from build123d import *

# Parameters (mm, degrees)
PAD_DEPTH       = 100
POCKET_DEPTH    = 2
POCKET001_DEPTH = 3


with BuildPart() as part:
    # Sketch → Pad (new body)
    with BuildSketch(Plane.XZ):
        Polygon((0, 0), (-15, 0), (-15, 1.5), (-14, 1.5), (-14, 5.5), (-17.5, 6.5), (-17.5, 7.5), (-12.5, 7.5), (-12.5, 1.5), (0, 1.5), (12.5, 1.5), (12.5, 7.5), (17.5, 7.5), (17.51485, 6.5), (14, 5.5), (14, 1.5), (15, 1.5), (15, 0), align=None)
    extrude(amount=PAD_DEPTH)

    # Sketch001 (on Face10 of Pad) → Pocket (cut)
    with BuildSketch(Plane(origin=(0, 0, 1.5), x_dir=(-1, 0, 0), z_dir=(0, 0, 1))):
        with BuildLine():
            ThreePointArc((2.5, 4.187631), (0, 6.687631), (-2.5, 4.187631))
            Line((-2.5, 4.187631), (-2.5, -0.812369))
            ThreePointArc((-2.5, -0.812369), (0, -3.312369), (2.5, -0.812369))
            Line((2.5, 4.187631), (2.5, -0.812369))
        make_face()
        with BuildLine():
            ThreePointArc((2.50462, 16.68763), (0.00462, 19.18763), (-2.49538, 16.68763))
            Line((-2.49538, 16.68763), (-2.49538, 11.68763))
            ThreePointArc((-2.49538, 11.68763), (0.00462, 9.18763), (2.50462, 11.68763))
            Line((2.50462, 16.68763), (2.50462, 11.68763))
        make_face()
        with BuildLine():
            ThreePointArc((2.509241, 29.187629), (0.009241, 31.687629), (-2.490759, 29.187629))
            Line((-2.490759, 29.187629), (-2.490759, 24.187629))
            ThreePointArc((-2.490759, 24.187629), (0.009241, 21.687629), (2.509241, 24.187629))
            Line((2.509241, 29.187629), (2.509241, 24.187629))
        make_face()
        with BuildLine():
            ThreePointArc((2.513861, 41.687629), (0.013861, 44.187629), (-2.486139, 41.687629))
            Line((-2.486139, 41.687629), (-2.486139, 36.687629))
            ThreePointArc((-2.486139, 36.687629), (0.013861, 34.187629), (2.513861, 36.687629))
            Line((2.513861, 41.687629), (2.513861, 36.687629))
        make_face()
        with BuildLine():
            ThreePointArc((2.518482, 54.187628), (0.018482, 56.687628), (-2.481518, 54.187628))
            Line((-2.481518, 54.187628), (-2.481518, 49.187628))
            ThreePointArc((-2.481518, 49.187628), (0.018482, 46.687628), (2.518482, 49.187628))
            Line((2.518482, 54.187628), (2.518482, 49.187628))
        make_face()
        with BuildLine():
            ThreePointArc((2.523102, 66.687627), (0.023102, 69.187627), (-2.476898, 66.687627))
            Line((-2.476898, 66.687627), (-2.476898, 61.687627))
            ThreePointArc((-2.476898, 61.687627), (0.023102, 59.187627), (2.523102, 61.687627))
            Line((2.523102, 66.687627), (2.523102, 61.687627))
        make_face()
        with BuildLine():
            ThreePointArc((2.527723, 79.187626), (0.027723, 81.687626), (-2.472277, 79.187626))
            Line((-2.472277, 79.187626), (-2.472277, 74.187626))
            ThreePointArc((-2.472277, 74.187626), (0.027723, 71.687626), (2.527723, 74.187626))
            Line((2.527723, 79.187626), (2.527723, 74.187626))
        make_face()
        with BuildLine():
            ThreePointArc((2.532343, 91.687625), (0.032343, 94.187625), (-2.467657, 91.687625))
            Line((-2.467657, 91.687625), (-2.467657, 86.687625))
            ThreePointArc((-2.467657, 86.687625), (0.032343, 84.187625), (2.532343, 86.687625))
            Line((2.532343, 91.687625), (2.532343, 86.687625))
        make_face()
        with BuildLine():
            ThreePointArc((2.536964, 104.187624), (0.036964, 106.687624), (-2.463036, 104.187624))
            Line((-2.463036, 104.187624), (-2.463036, 99.187624))
            ThreePointArc((-2.463036, 99.187624), (0.036964, 96.687624), (2.536964, 99.187624))
            Line((2.536964, 104.187624), (2.536964, 99.187624))
        make_face()
        with BuildLine():
            ThreePointArc((2.541584, 116.687623), (0.041584, 119.187623), (-2.458416, 116.687623))
            Line((-2.458416, 116.687623), (-2.458416, 111.687623))
            ThreePointArc((-2.458416, 111.687623), (0.041584, 109.187623), (2.541584, 111.687623))
            Line((2.541584, 116.687623), (2.541584, 111.687623))
        make_face()
    extrude(amount=-POCKET_DEPTH, mode=Mode.SUBTRACT)

    # Sketch001 (on Face10 of Pad) → Pocket001 (cut)
    with BuildSketch(Plane(origin=(0, 0, 1.5), x_dir=(-1, 0, 0), z_dir=(0, 0, 1))):
        with BuildLine():
            ThreePointArc((2.5, 4.187631), (0, 6.687631), (-2.5, 4.187631))
            Line((-2.5, 4.187631), (-2.5, -0.812369))
            ThreePointArc((-2.5, -0.812369), (0, -3.312369), (2.5, -0.812369))
            Line((2.5, 4.187631), (2.5, -0.812369))
        make_face()
        with BuildLine():
            ThreePointArc((2.50462, 16.68763), (0.00462, 19.18763), (-2.49538, 16.68763))
            Line((-2.49538, 16.68763), (-2.49538, 11.68763))
            ThreePointArc((-2.49538, 11.68763), (0.00462, 9.18763), (2.50462, 11.68763))
            Line((2.50462, 16.68763), (2.50462, 11.68763))
        make_face()
        with BuildLine():
            ThreePointArc((2.509241, 29.187629), (0.009241, 31.687629), (-2.490759, 29.187629))
            Line((-2.490759, 29.187629), (-2.490759, 24.187629))
            ThreePointArc((-2.490759, 24.187629), (0.009241, 21.687629), (2.509241, 24.187629))
            Line((2.509241, 29.187629), (2.509241, 24.187629))
        make_face()
        with BuildLine():
            ThreePointArc((2.513861, 41.687629), (0.013861, 44.187629), (-2.486139, 41.687629))
            Line((-2.486139, 41.687629), (-2.486139, 36.687629))
            ThreePointArc((-2.486139, 36.687629), (0.013861, 34.187629), (2.513861, 36.687629))
            Line((2.513861, 41.687629), (2.513861, 36.687629))
        make_face()
        with BuildLine():
            ThreePointArc((2.518482, 54.187628), (0.018482, 56.687628), (-2.481518, 54.187628))
            Line((-2.481518, 54.187628), (-2.481518, 49.187628))
            ThreePointArc((-2.481518, 49.187628), (0.018482, 46.687628), (2.518482, 49.187628))
            Line((2.518482, 54.187628), (2.518482, 49.187628))
        make_face()
        with BuildLine():
            ThreePointArc((2.523102, 66.687627), (0.023102, 69.187627), (-2.476898, 66.687627))
            Line((-2.476898, 66.687627), (-2.476898, 61.687627))
            ThreePointArc((-2.476898, 61.687627), (0.023102, 59.187627), (2.523102, 61.687627))
            Line((2.523102, 66.687627), (2.523102, 61.687627))
        make_face()
        with BuildLine():
            ThreePointArc((2.527723, 79.187626), (0.027723, 81.687626), (-2.472277, 79.187626))
            Line((-2.472277, 79.187626), (-2.472277, 74.187626))
            ThreePointArc((-2.472277, 74.187626), (0.027723, 71.687626), (2.527723, 74.187626))
            Line((2.527723, 79.187626), (2.527723, 74.187626))
        make_face()
        with BuildLine():
            ThreePointArc((2.532343, 91.687625), (0.032343, 94.187625), (-2.467657, 91.687625))
            Line((-2.467657, 91.687625), (-2.467657, 86.687625))
            ThreePointArc((-2.467657, 86.687625), (0.032343, 84.187625), (2.532343, 86.687625))
            Line((2.532343, 91.687625), (2.532343, 86.687625))
        make_face()
        with BuildLine():
            ThreePointArc((2.536964, 104.187624), (0.036964, 106.687624), (-2.463036, 104.187624))
            Line((-2.463036, 104.187624), (-2.463036, 99.187624))
            ThreePointArc((-2.463036, 99.187624), (0.036964, 96.687624), (2.536964, 99.187624))
            Line((2.536964, 104.187624), (2.536964, 99.187624))
        make_face()
        with BuildLine():
            ThreePointArc((2.541584, 116.687623), (0.041584, 119.187623), (-2.458416, 116.687623))
            Line((-2.458416, 116.687623), (-2.458416, 111.687623))
            ThreePointArc((-2.458416, 111.687623), (0.041584, 109.187623), (2.541584, 111.687623))
            Line((2.541584, 116.687623), (2.541584, 111.687623))
        make_face()
    extrude(amount=-POCKET001_DEPTH, mode=Mode.SUBTRACT)


solid = part.part
Could you check a few things on this model? Use its own coordinates, in mm. A direction names the side the tool comes from. Give positions to 0.01 mm unless a question says otherwise; leave off trailing zeros. Order: outer loops, then holes, each group sorted by start corner. A loop starts at its lowest first (then second) coordinate and runs counter-clockwise, first axis right, second up.
1. I need wall thicknesses on L1, parallel to X at y = -87, z = 4.5; L2, parallel to X at y = -78.5, z = 0.75; L3, parallel to Z at x = -5, y = -31. Which ranges of each line are inside material? Lowest first, please.
2. We'd pull the mould along Y, two halves only. Please class faces 4 (the cylindrical face through (0.02, -96.69, 0.76)), 5 (the flat face through (-12.5, -49, 5)), 6 (the cylindrical face through (-0.073, -56.687, 0.76)): pulls with the +Y half, pulls with the -Y half, needs draft (parallel to the pull), parting line crosses it, or undercut.
3. For faces 1 (the cylindrical face through (0.02, -84.19, 0.76)), 2 (the flat face through (11, 0, 1)), 3 (the flat face through (-15.726, -49.3, 5.993)), which set-ups out of +Z, -Z, +X, -X, +Y, -Y let a thin tool reach every point of the face, with its end or its side?
4. Suppose I cut it at A-A (z = 2.5). List the corners of the cut face in (x, y) for me.
5. Suppose I cut it at B-B (x = 0.5). Give the number of separate pieces and of enclosed holes in the cut face, plus the area to 3 significant figures.
6. Will these pins go through, and if not, where does the flat tip stop? P1, Ø1.6, axis at y = -65.5, z = 0.5, coming from the -X side; P2, Ø12, axis at x = -2.5, y = -47, coming from the +Z side; P3, Ø1.2, axis at y = -33, z = 4, coming from the -X side; P4, Ø5, axis at x = 5, y = -21, coming from the -Z side.
7. Suppose I cut it at C-C (x = -5). List the corners of the cut face in (y, z) for me, plus the area to 3 significant figures.
Solved:
1. L1: x = -14 to -12.5, 12.5 to 14
1. L2: x = -15 to -2.53, 2.47 to 15
1. L3: z = 0 to 1.5
2. face 4: pulls with the -Y half
2. face 5: needs draft
2. face 6: undercut
3. face 1: +Z, -Z
3. face 2: +Z, -Z, +X, -X, +Y
3. face 3: -X, +Y, -Y
4. outline: (-14, -100) - (-12.5, -100) - (-12.5, 0) - (-14, 0) - close; (12.5, -100) - (14, -100) - (14, 0) - (12.5, 0) - close
5. separate pieces: 8
5. enclosed holes: 0
5. area: 31.3 mm2
6. P1: stops at x = -15
6. P2: stops at z = 1.5
6. P3: stops at x = -14
6. P4: stops at z = 0
7. outline: (-100, 0) - (0, 0) - (0, 1.5) - (-100, 1.5) - close
7. area: 150 mm2
